Read the model definition and answer for the solid it produces. Units are mm, in the model's axes. A direction names the side the tool comes from. Give positions to 0.01 mm unless a question says otherwise; leave off trailing zeros. Order: outer loops, then holes, each group sorted by start corner. A loop starts at its lowest first (then second) coordinate and runs counter-clockwise, first axis right, second up. Notation, with made-up numbers: M -4,-4 L 1,-4 A12 ccw 1,15 Z; hole C 86,-32 d1. An arc over 180 degrees is marked long. One line per item, written item: value. Start each with the question number.
from build123d import *

# Parameters (mm, degrees)
SKETCH_1_R      = 1.45
EXTRUDE_1_DEPTH = 3


with BuildPart() as part:
    # 草图1 → 凸台-拉伸1 (new body)
    # profile 1 of 3: a face of its own
    with BuildSketch(Plane(origin=(0, 0, 0), x_dir=(1, 0, 0), z_dir=(0, 1, 0))):
        with BuildLine():
            Line((20, 0), (5, 0))
            ThreePointArc((5, 0), (1.464466094, -1.464466094), (0, -5))
            Line((0, -5), (0, -45))
            Line((0, -45), (2.5, -45))
            Line((2.5, -45), (9.75, -45))
            Line((9.75, -45), (9.75, -41))
            Line((9.75, -41), (11, -41))
            Line((11, -41), (11, -38))
            Line((11, -38), (14, -38))
            Line((14, -38), (14, -41))
            Line((14, -41), (15.25, -41))
            Line((15.25, -41), (15.25, -45))
            Line((15.25, -45), (22.5, -45))
            Line((22.5, -45), (25, -45))
            Line((25, -45), (25, -5))
            ThreePointArc((25, -5), (23.535533906, -1.464466094), (20, 0))
        make_face()
        with Locations(Location((12.5, -5, 0), (0, 0, 270))):
            Circle(SKETCH_1_R, mode=Mode.SUBTRACT)
    # profile 2 of 3: a face of its own
    with BuildSketch(Plane(origin=(0, 0, 0), x_dir=(1, 0, 0), z_dir=(0, 1, 0))):
        Polygon((22.5, -48), (22.5, -45), (15.25, -45), (14, -45), (14, -48), align=None)
    # profile 3 of 3: a face of its own
    with BuildSketch(Plane(origin=(0, 0, 0), x_dir=(1, 0, 0), z_dir=(0, 1, 0))):
        Polygon((9.75, -45), (2.5, -45), (2.5, -48), (11, -48), (11, -45), align=None)
    extrude(amount=EXTRUDE_1_DEPTH)


solid = part.part
Q1. Find section B-B, the plane x = 12.5. Give the vertices of the cut face in (y, z).
Q2. Each of these flat-tipped pins is pushed along its axis until it touches: pin 1 (0.9 mm diameter, centred on y = 2, z = 47, fed in from +X); pin 2 (0.9 mm diameter, centred on y = 2, z = 46, fed in from -X). Where does it stop, or does it pass through?
Q3. Determine the mould class of faces 4 (the flat face through (12, 1, 38)), 5 (the flat face through (25, 1, 25)), 6 (the flat face through (15, 1, 45)) for opening direction Z: released by +Z, released by -Z, zero draft, split by the parting line, or undercut.
Q4. Find section C-C, the plane x = 23. Give the vertices of the cut face in (y, z), then the cut area to 3 significant figures.
Q5. A tool of negligible diameter and unlimited length cuts with its end or side. For faces 1 (the flat face through (24, 1, 45)), 2 (the flat face through (15.25, 1, 43)), 3 (the flat face through (1, 1, 45)), from which of +Z, -Z, +X, -X, +Y, -Y can it reach the whole face along a straight path? Write none if from no direction.
Q6. Find section A-A, the plane y = 0.7. Give the vertices of the cut face in (x, z).
Q7. Consider probe 1 along X at (y, z) = (1.4, 5); probe 2 along X at (y, z) = (2.1, 42.5); probe 3 along Z at (x, y) = (14.25, 0.85). Determine where each line is inside the solid, lowest interval first.
Evaluation:
1. outline: M 0,0 L 3,0 L 3,3.55 L 0,3.55 Z; M 0,6.45 L 3,6.45 L 3,38 L 0,38 Z
2. pin 1: x = 22.5
2. pin 2: x = 2.5
3. face 4: released by +Z
3. face 5: zero draft
3. face 6: undercut
4. outline: M 0,1 L 3,1 L 3,45 L 0,45 Z
4. area: 132 mm2
5. face 1: +Z, +X, +Y, -Y
5. face 2: +Y, -Y
5. face 3: +Z, -X, +Y, -Y
6. outline: M 0,5 A5 ccw 5,0 L 20,0 A5 ccw 25,5 L 25,45 L 22.5,45 L 22.5,48 L 14,48 L 14,45 L 15.25,45 L 15.25,41 L 14,41 L 14,38 L 11,38 L 11,41 L 9.75,41 L 9.75,45 L 11,45 L 11,48 L 2.5,48 L 2.5,45 L 0,45 Z; hole C 12.5,5 d2.9
7. probe 1: 0 to 11.05, 13.95 to 25
7. probe 2: 0 to 9.75, 15.25 to 25
7. probe 3: 0 to 41, 45 to 48
